Check sheet for the modelled part. Datum: model origin and axes. Units: mm. Round coordinates to 2 decimals unless told otherwise and drop trailing zeros. Order: outer loops, then holes, each group sorted by start corner. A loop starts at its lowest first (then second) coordinate and runs counter-clockwise, first axis right, second up.
Q1. Cross-section at D-D on y = -47.25. Record the cut outline in (x, z).
Q2. Depth check by flat-ended pin: P1, Ø5, axis at x = 74.43, y = -52.25, coming from the -Z side; P2, Ø1, axis at y = -53, z = 4.5, coming from the -X side. Enter the tip coordinate at first touch or a pass-through.
Q3. Scan lines: probe 1 along X at (y, z) = (-52.75, 3.5); probe 2 along X at (y, z) = (-50.5, 5.75); probe 3 along Y at (x, z) = (76, 5.25). Record each from-to range of solid material in increasing order.
Q4. Mould release check, pull along X, two halves, no side actions. Record for faces 1 (the cylindrical face through (84.43, -52.47, 3.13)), 2 (the cylindrical face through (-60.566, -52.026, 3.131)), 3 (the cylindrical face through (77.365, -53.462, 3.131)): +X half, -X half, draft (parallel to the pull), parting line (faces both ways), or undercut.
Q5. Cross-section at C-C on y = -59.75. Record the cut outline in (x, z).
Q6. Cross-section at A-A on x = 10.5. Record the cut outline in (y, z).
Q7. Cross-section at B-B on z = 3.5. Record the cut outline in (x, y) (3 decimals), then the cut area to 3 significant figures.
from build123d import *

# Parameters (mm, degrees)
F2_DEPTH = 6.35
F1_R     = 3.175
F3_DEPTH = 6.351


with BuildPart() as f2:
    # F0 (on Top) → F2 (new body)
    with BuildSketch(Plane.XY):
        with BuildLine():
            Line((74.432049, -42.245469), (-50.567951, -42.245469))
            ThreePointArc((-50.567951, -42.245469), (-60.567951, -52.245469), (-50.567951, -62.245469))
            Line((-50.567951, -62.245469), (74.432049, -62.245469))
            ThreePointArc((74.432049, -62.245469), (84.432049, -52.245469), (74.432049, -42.245469))
        make_face()
    extrude(amount=F2_DEPTH)

    # F1 (on Top) → F3 (cut, through all)
    with BuildSketch(Plane.XY):
        with Locations((-50.567951, -52.245469)):
            Circle(F1_R)
        with Locations((74.432049, -52.245469)):
            Circle(F1_R)
        with Locations((11.932049, -52.245469)):
            Circle(F1_R)
    extrude(amount=F3_DEPTH, mode=Mode.SUBTRACT)


solid = f2.part
Results found:
1. outline: (-59.23, 0) - (83.09, 0) - (83.09, 6.35) - (-59.23, 6.35) - close
2. P1: passes through
2. P2: stops at x = -60.56
3. probe 1: x = -60.56 to -53.7, -47.43 to 8.8, 15.07 to 71.3, 77.57 to 84.42
3. probe 2: x = -60.41 to -53.22, -47.92 to 9.28, 14.58 to 71.78, 77.08 to 84.28
3. probe 3: y = -62.12 to -55.01, -49.48 to -42.37
4. face 1: +X half
4. face 2: -X half
4. face 3: undercut
5. outline: (-57.18, 0) - (81.04, 0) - (81.04, 6.35) - (-57.18, 6.35) - close
6. outline: (-62.25, 0) - (-55.08, 0) - (-55.08, 6.35) - (-62.25, 6.35) - close; (-49.41, 0) - (-42.25, 0) - (-42.25, 6.35) - (-49.41, 6.35) - close
7. outline: (-50.568, -62.245) - (74.432, -62.245) arc R10 ccw to (74.432, -42.245) - (-50.568, -42.245) arc R10 ccw to start; hole circle Ø6.35 at (-50.568, -52.245); hole circle Ø6.35 at (11.932, -52.245); hole circle Ø6.35 at (74.432, -52.245)
7. area: 2,720 mm2
